Part print with two shaded views. Sizes in mm from the minimum x, y, z corner. A direction names the side the tool comes from. Coordinates: 2 decimals unless noted, no trailing zeros. Write each loop counter-clockwise with the first axis right and the second up, starting at its lowest first coordinate (ties: lowest second). Pieces come first, ordered by that corner, then holes.
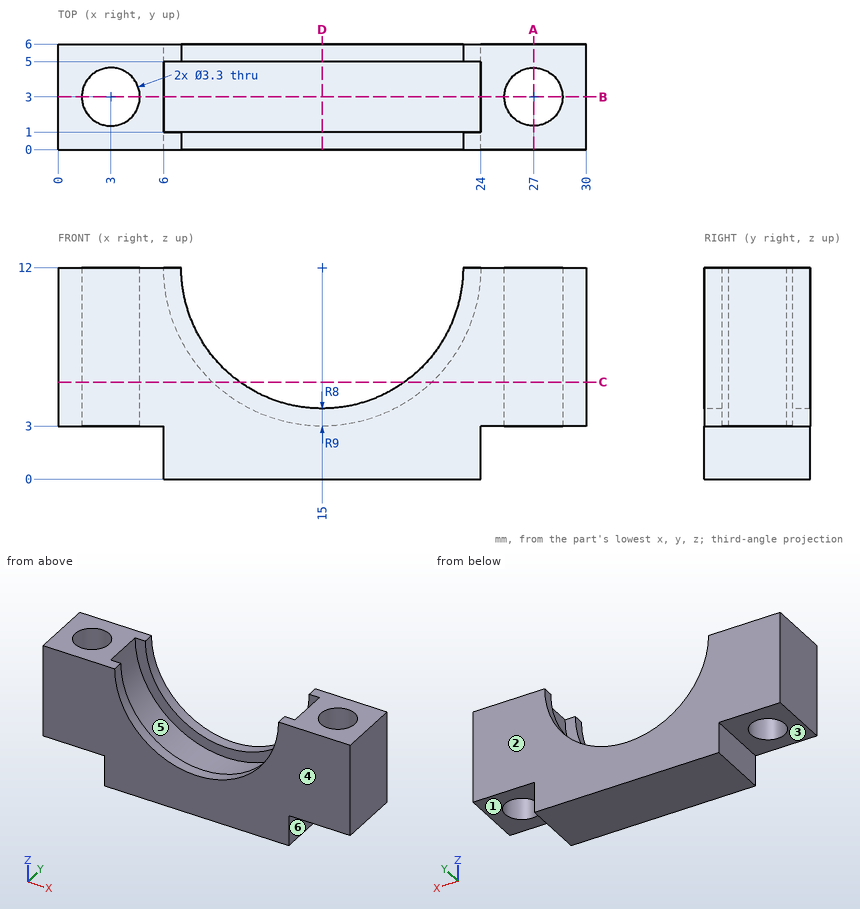
(1) Slice it at B-B, the plane y = 3. List the corners of the cut face in (x, z).
(2) 3-axis set-ups, long thin cutter, end or side, ignore diameter. For the marked faces 1, 2 and 3: which of +Z, -Z, +X, -X, +Y, -Y reach the whole face in a straight line?
(3) Probe L1, parallel to Y at x = 3, z = 8.75; L2, parallel to Y at x = 10.5, z = 4.75; L3, parallel to X at y = 3.25, z = 11.25. List the from-to ranges inside material, lowest first.
(4) Slice it at A-A, the plane x = 27. List the corners of the cut face in (y, z), and give its area (3 significant figures).
(5) Two-plate mould, pull along Y, no slides. Class the marked faces 4, 5 and 6: pulls with the +Y half, pulls with the -Y half, needs draft (parallel to the pull), parting line crosses it, or undercut.
(6) Flat gauge pins, fed straight in: P1, Ø2.5, axis at y = 4, z = 1, coming from the -X side; P2, Ø1.5, axis at y = 4.5, z = 2, coming from the +X side. Where does each tip first touch, or does it go through?
(7) Slice it at C-C, the plane z = 5.5. List the corners of the cut face in (x, y), and give its area (3 significant figures).
(8) Slice it at D-D, the plane x = 15. List the corners of the cut face in (y, z).
Results:
1. outline: (0, 3) - (1.35, 3) - (1.35, 12) - (0, 12) - close; (4.65, 3) - (6, 3) - (6, 0) - (24, 0) - (24, 3) - (25.35, 3) - (25.35, 12) - (24, 12) arc R9 cw to (6, 12) - (4.65, 12) - close; (28.65, 3) - (30, 3) - (30, 12) - (28.65, 12) - close
2. face 1: -Z, +X, +Y, -Y
2. face 2: +Z, -Z, +X, -X, +Y
2. face 3: -Z, -X, +Y, -Y
3. L1: y = 0 to 1.35, 4.65 to 6
3. L2: y = 0 to 1, 5 to 6
3. L3: x = 0 to 1.37, 4.63 to 6.03, 23.97 to 25.37, 28.63 to 30
4. outline: (0, 3) - (1.35, 3) - (1.35, 12) - (0, 12) - close; (4.65, 3) - (6, 3) - (6, 12) - (4.65, 12) - close
4. area: 24.3 mm2
5. face 4: pulls with the -Y half
5. face 5: undercut
5. face 6: needs draft
6. P1: stops at x = 6
6. P2: stops at x = 24
7. outline: (0, 0) - (10.34, 0) - (10.34, 1) - (8.78, 1) - (8.78, 5) - (10.34, 5) - (10.34, 6) - (0, 6) - close; (19.66, 0) - (30, 0) - (30, 6) - (19.66, 6) - (19.66, 5) - (21.22, 5) - (21.22, 1) - (19.66, 1) - close; hole circle Ø3.3 at (3, 3); hole circle Ø3.3 at (27, 3)
7. area: 94.4 mm2
8. outline: (0, 0) - (6, 0) - (6, 4) - (5, 4) - (5, 3) - (1, 3) - (1, 4) - (0, 4) - close
